Verification items for the finished model (mm, model axes). A direction names the side the tool comes from. Give positions to 0.01 mm unless a question says otherwise; leave off trailing zeros. Order: outer loops, then holes, each group sorted by start corner. A loop starts at its lowest first (then second) coordinate and runs counter-clockwise, first axis right, second up. Notation, with made-up numbers: (79, -26.75) -> (88, -26.75) arc R28 cw to (88, -0.75) -> close; hole circle Ø8 at (79.5, -23.75). An arc over 180 degrees is marked (long way). One line per question, with ' | ' between items. Start each with the question number.
Q1. Go/stop test with flat-tipped pins: pin 1 (4 mm diameter, centred on x = 2, y = -58.5, fed in from -Z); pin 2 (2 mm diameter, centred on y = -58.5, z = -3.5, fed in from -X); pin 3 (3 mm diameter, centred on x = 1, y = -55.5, fed in from +Z). Record where each tip stops, or that it passes through.
Q2. Mould release check, pull along X, two halves, no side actions. Record for faces 1 (the conical face through (-0.381, 1.787, -0.12)), 2 (the flat face through (-0.1, 0, 3.3)), 3 (the cylindrical face through (5, 3, 0)), 4 (the flat face through (2.155, 4.521, -1.267)): released by +X, released by -X, zero draft, split by the parting line, or undercut.
Q3. Access from +Z, -Z, +X, -X, +Y, -Y to the whole of each face (thin tool, end or side, straight path). Record for faces 5 (the flat face through (-2, 6, 2)), 6 (the flat face through (-2.175, 4.521, -1.233)), 7 (the cylindrical face through (0.9, -34.02, 2.86)).
Q4. Section check A-A on y = -16.5. Record the cut outline in (x, z).
Q5. Material ranges on probe 1 along Z at (x, y) = (-2.25, -12); probe 2 along Y at (x, z) = (-2.5, -2), recorded low to high. Write a range as [from, to].
from build123d import *

# Parameters (mm, degrees)
ESQUISSE1_R             = 3
TIGE_DEPTH              = 70
CHANFREIN_D_ENTR_E_SIZE = 1
HEXAGONE_DEPTH          = 3


with BuildPart() as part:
    # Esquisse1 → Tige (new body)
    with BuildSketch(Plane(origin=(0, 0, 0), x_dir=(1, 0, 0), z_dir=(0, 1, 0))):
        with Locations(Location((0, 0, 0), (0, 0, 270))):
            Circle(ESQUISSE1_R)
    extrude(amount=-TIGE_DEPTH)

    # Chanfrein d_entr_e
    chanfrein_d_entr_e_edges = [part.edges().sort_by_distance(p)[0] for p in [
        (0, -70, -3),
    ]]
    chamfer(chanfrein_d_entr_e_edges, length=CHANFREIN_D_ENTR_E_SIZE)

    # Esquisse2 → T_te (revolve)
    with BuildSketch(Plane.XY, mode=Mode.PRIVATE) as t_te_sk:
        with BuildLine():
            Line((2.5, 6), (2.5, 3))
            Line((2.5, 3), (0, 1.556624327))
            Line((0, 1.556624327), (0, 0))
            Line((0, 0), (5, 0))
            Line((5, 0), (5, 5.4))
            ThreePointArc((5, 5.4), (4.824264069, 5.824264069), (4.4, 6))
            Line((4.4, 6), (2.5, 6))
        make_face()
    revolve(t_te_sk.sketch.rotate(Axis((0, 6, 0), (0, -1, 0)), 180), axis=Axis((0, 6, 0), (0, -1, 0)))

    # Esquisse3 → Hexagone (cut)
    with BuildSketch(Plane(origin=(0, 6, -3), x_dir=(1, 0, 0), z_dir=(0, -1, 0))):
        Polygon((1.443375673, 5.5), (-1.443375673, 5.5), (-2.886751346, 3), (-1.443375673, 0.5), (1.443375673, 0.5), (2.886751346, 3), align=None)
    extrude(amount=HEXAGONE_DEPTH, mode=Mode.SUBTRACT)


solid = part.part
Filled in:
1) pin 1: z = -3 | pin 2: x = -1.66 | pin 3: z = 3
2) face 1: undercut | face 2: zero draft | face 3: split by the parting line | face 4: undercut
3) face 5: +Z, -Z, +X, -X, +Y | face 6: +Y | face 7: -Y
4) outline: circle Ø6 at (0, 0)
5) probe 1: [-1.98, 1.98] | probe 2: [0, 6]
